Autodesk Inventor part; units mm, degrees
ref_plane "YZ Plane" through (0, 0, 0) normal (1, 0, 0) x (0, 1, 0)
ref_plane "XZ Plane" through (0, 0, 0) normal (0, 1, 0) x (-1, 0, 0)
ref_plane "XY Plane" through (0, 0, 0) normal (0, 0, 1) x (1, 0, 0)
sketch "Sketch1" plane through (0, 0, 0) normal (0, 1, 0) x (-1, 0, 0)
  line L0 (0, 0) -> (124.865, 0)
  line L1 (124.865, 0) -> (124.865, -120)
  line L2 (124.865, -120) -> (0, -120)
  line L3 (0, -120) -> (0, 0)
  dimension "d0" = 124.865
  dimension "d1" = 120
extrude "Extrusion1" add sketch "Sketch1" along normal blind 3.5
sketch "Sketch2" plane through (0, 0, 0) normal (0, -1, 0) x (1, 0, 0)
  circle A0 centre (-117.615, -60) radius 1.75
  circle A1 centre (-7.25, -60) radius 1.75
  line L0 (-124.865, 0) -> (-124.865, -120)
  line L1 (0, 0) -> (-124.865, 0)
  line L2 (0, -120) -> (0, 0)
  dimension "d4" = 3.5
  dimension "d5" = 3.5
  dimension "d6" = 7.25
  dimension "d7" = 60
  dimension "d8" = 7.25
  dimension "d9" = 60
hole "Hole1" at (-7.25, 0, -60) at (-117.615, 0, -60) direction (0, 1, 0) diameter 3.5 end through all countersink diameter 5.5 countersink angle 90
sketch "Sketch3" plane through (0, 0, -120) normal (0, 0, -1) x (-1, 0, 0)
  line L0 (73.933, -5) -> (73.933, 0)
  line L1 (70.433, 0) -> (70.433, -5)
  line L2 (50.933, 0) -> (50.933, -5)
  line L3 (54.433, -5) -> (54.433, 0)
  arc A0 (54.433, -5) -> (70.433, -5) centre (62.433, -5) ccw
  arc A1 (50.933, -5) -> (73.933, -5) centre (62.433, -5) ccw
  line L4 (73.933, 0) -> (73.933, 3.5)
  line L5 (0, 3.5) -> (124.865, 3.5)
  line L6 (50.933, 0) -> (50.933, 3.5)
  line L7 (73.933, 3.5) -> (50.933, 3.5)
  line L8 (70.433, 0) -> (54.433, 0)
  line L9 (124.865, 0) -> (0, 0)
  dimension "d22" = 3.5
  dimension "d24" = 3.5
extrude "Extrusion2" add sketch "Sketch3" against normal blind 120
sketch "Sketch4" plane through (0, 3.5, -120) normal (0, 0, -1) x (-1, 0, 0)
  line L0 (124.865, -3.5) -> (124.865, 0)
  line L1 (70.433, -3.5) -> (70.433, -8.5)
  line L2 (54.433, -3.5) -> (54.433, -8.5)
  arc A0 (54.433, -8.5) -> (70.433, -8.5) centre (62.433, -8.5) ccw
  line L3 (70.433, -3.5) -> (70.433, 0)
  line L4 (70.433, 0) -> (54.433, 0)
  line L5 (54.433, 0) -> (54.433, -3.5)
  point P0 (0, -3.5)
extrude "Extrusion3" cut sketch "Sketch4" against normal blind 120
sketch "Sketch5" plane through (0, 3.5, 0) normal (0, 1, 0) x (1, 0, 0)
  line L0 (0, 120) -> (0, 0)
  arc A0 (0, 120) -> (0, 0) centre (138.5716, 60) ccw
  line L1 (-70.433, 120) -> (-124.865, 120)
  arc A1 (-124.865, 0) -> (-124.865, 120) centre (-262.4456, 60) ccw
extrude "Extrusion4" add sketch "Sketch5" along normal blind 5
sketch "Sketch6" plane through (0, 3.5, 0) normal (0, 1, 0) x (1, 0, 0)
  line L0 (-124.865, 120) -> (-124.865, 0)
  arc A0 (-124.865, 0) -> (-124.865, 120) centre (-263.4366, 60) ccw
  point P0 (0, 0)
extrude "Extrusion5" add sketch "Sketch6" along normal blind 5
hole "Hole3" at (-117.615, 3.5, -60) direction (0, 1, 0) diameter 3.5 end through all
hole "Hole4" at (-7.2464, 3.5, -59.9915) direction (0, 1, 0) diameter 3.5 end through all
fillet "Fillet2" radius 5 2 edges at (-50.933, 0, -60) (-73.933, 0, -60)
chamfer "Chamfer1" distance 2 angle 45 12 edges at (-124.865, 0, -60) (0, 0, -60) (-62.433, -16.5, -120) (-49.4686, -1.4644, -120) (-22.9665, 0, -120) (-75.3974, -1.4644, -120) (-101.8989, 0, -120) (-62.433, -16.5, 0) (-49.4686, -1.4644, 0) (-22.9665, 0, 0) (-75.3974, -1.4644, 0) (-101.8989, 0, 0)
properties part number "FinalBack"
Verification items for the finished model (mm, model axes). A direction names the side the tool comes from. Give positions to 0.01 mm unless a question says otherwise; leave off trailing zeros. Write each loop counter-clockwise with the first axis right and the second up, starting at its lowest first coordinate (ties: lowest second). Pieces come first, ordered by that corner, then holes. Notation, with made-up numbers: M 51,3.25 L 76,3.25 A14 cw 76,10.25 Z; hole C 8,-30.5 d1. An arc over 180 degrees is marked long. Write item = value, one per line.
(1) Draft check along Z on faces 4 (the face through (-75.36, -1.5, -59.19)), 5 (the face through (-74.793, -0.95, -1.208)), 6 (the face through (-6.58, 6.04, -61.61)), 7 (the face through (-6.58, 2.268, -61.617)). Enter one of: released by +Z, released by -Z, zero draft, split by the parting line, or undercut.
Found:
face_4 = zero draft
face_5 = released by +Z
face_6 = undercut
face_7 = undercut
(2) Sectioned sample at A-A (x = -31). Record the cut outline in (y, z), then the cut area to 3 significant figures.
Found:
outline = M 0,-118 L 2,-120 L 3.5,-120 L 3.5,0 L 2,0 L 0,-2 Z
area = 416 mm2
(3) Access from +Z, -Z, +X, -X, +Y, -Y to the whole of each face (thin tool, end or side, straight path). Record for faces 1 (the face through (-24, 0, -59)), 2 (the face through (-54.433, -1, -61)), 3 (the face through (-12.43, 5.96, -59.14)).
Found:
face_1 = +Z, -Z, +X, -Y
face_2 = +Z, -Z, +Y
face_3 = +Y
(4) Go/stop test with flat-tipped pins: pin 1 Ø12 at (y, z) = (-11, -43) entering from -X; pin 2 Ø2 at (y, z) = (-10.5, -77.5) entering from -X; pin 3 Ø6 at (y, z) = (-10, -75) entering from -X; pin 4 Ø9.5 at (y, z) = (0.5, -57.5) entering from +X. Record where each tip stops, or that it passes through.
Found:
pin_1 = -73.93
pin_2 = -73.02
pin_3 = -73.76
pin_4 = 0
(5) Material ranges on line 1 (Y direction, x = -101, z = -58.5); line 2 (X direction, y = 1.6, z = -60) (3 decimals); line 3 (X direction, y = -6.5, z = -104.5), recorded low to high.
Found:
line_1 = 0 to 3.5
line_2 = -124.465 to -119.365, -115.865 to -70.433, -54.433 to -9, -5.5 to -0.4
line_3 = -73.83 to -70.29, -54.57 to -51.03
